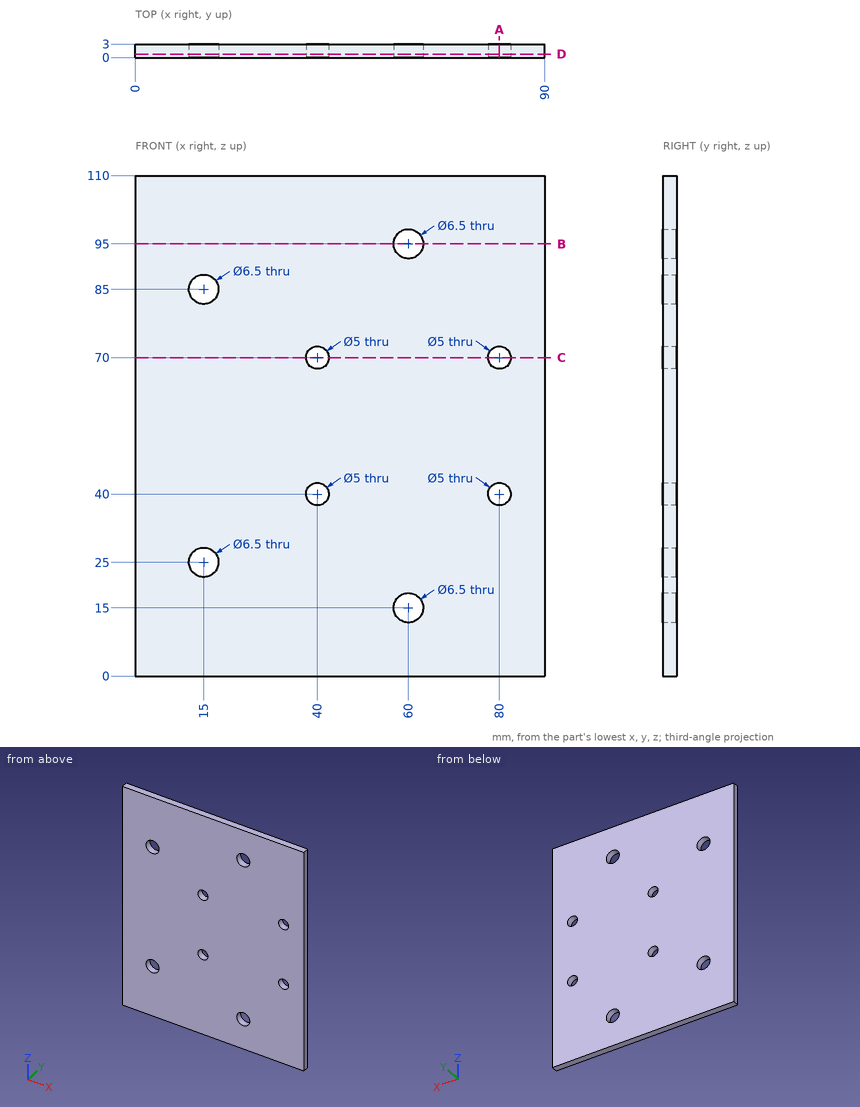
The figure shows three views and two pictorial views of one solid part (mm, origin at its lowest corner). Answer the questions. Give positions to 0.01 mm unless a question says otherwise; leave off trailing zeros. Write each loop counter-clockwise with the first axis right and the second up, starting at its lowest first coordinate (ties: lowest second). Pieces come first, ordered by that corner, then holes. Notation, with made-up numbers: (55, -23) - (110, -23) arc R22 cw to (110, -17) - close; hole circle Ø7 at (87.5, 55). An arc over 180 degrees is marked (long way). Use one line per item in the form item = value.
1. Consider L1, parallel to X at y = 2.1, z = 70; L2, parallel to X at y = 2.3, z = 85; L3, parallel to X at y = 1.55, z = 15. Determine where each line is inside the solid, lowest interval first.
Filled in:
L1 = 0 to 37.5, 42.5 to 77.5, 82.5 to 90
L2 = 0 to 11.75, 18.25 to 90
L3 = 0 to 56.75, 63.25 to 90
2. A cutting plane is placed at D-D (y = 0.75). State how many separate pieces and enclosed holes the cut face has, and give its area (3 significant figures).
Filled in:
separate_pieces = 1
enclosed_holes = 8
area = 9,690 mm^2
3. A cutting plane is placed at A-A (x = 80). Write down the section's boundary in (y, z), and give its area (3 significant figures).
Filled in:
outline = (0, 0) - (3, 0) - (3, 37.5) - (0, 37.5) - close; (0, 42.5) - (3, 42.5) - (3, 67.5) - (0, 67.5) - close; (0, 72.5) - (3, 72.5) - (3, 110) - (0, 110) - close
area = 300 mm^2
4. A cutting plane is placed at C-C (z = 70). Write down the section's boundary in (x, y).
Filled in:
outline = (0, 0) - (37.5, 0) - (37.5, 3) - (0, 3) - close; (42.5, 0) - (77.5, 0) - (77.5, 3) - (42.5, 3) - close; (82.5, 0) - (90, 0) - (90, 3) - (82.5, 3) - close
5. A cutting plane is placed at B-B (z = 95). Write down the section's boundary in (x, y).
Filled in:
outline = (0, 0) - (56.75, 0) - (56.75, 3) - (0, 3) - close; (63.25, 0) - (90, 0) - (90, 3) - (63.25, 3) - close
6. This flat-tipped pin is pushed along its axis until it touches: pin 1 Ø8.5 at (x, z) = (60, 95) entering from +Y. Where does it stop, or does it pass through?
Filled in:
pin_1 = 3
